```python
from build123d import *

# Parameters (mm, degrees)
BASPROSKE_W        = 9
BASPROSKE_H        = 11
TOOTHCUT_DEPTH     = 18.972200756
TEETHCUTS_COUNT    = 20
TEETHCUTS_ANGLE    = 342
BORSKE_R           = 3.5
BORE_DEPTH         = 50.0000508
SKETCH1_R          = 1.1
CUT_EXTRUDE1_DEPTH = 18.852389344


with BuildPart() as part:
    # BasProSke → Base-Revolve (revolve)
    with BuildSketch(Plane(origin=(0, 0, 0), x_dir=(1, 0, 0), z_dir=(0, 1, 0)), mode=Mode.PRIVATE) as base_revolve_sk:
        with Locations((4.5, 5.5)):
            Rectangle(BASPROSKE_W, BASPROSKE_H)
    revolve(base_revolve_sk.sketch.rotate(Axis((-10, 0, 0), (1, 0, 0)), 180), axis=Axis((-10, 0, 0), (1, 0, 0)))

    # TooCutSke → ToothCut (cut, through all)
    with BuildSketch(Plane(origin=(0, 0, 0), x_dir=(0, 0, -1), z_dir=(1, 0, 0))):
        with BuildLine():
            ThreePointArc((0.499924007, 8.734705318), (0, 8.749), (-0.499924007, 8.734705318))
            ThreePointArc((-0.499924007, 8.734705318), (-0.824302243, 9.905497836), (-1.485192705, 10.924909509))
            ThreePointArc((-1.485192705, 10.924909509), (0, 11.0254), (1.485192705, 10.924909509))
            ThreePointArc((1.485192705, 10.924909509), (0.824302243, 9.905497836), (0.499924007, 8.734705318))
        make_face()
    toothcut = extrude(amount=TOOTHCUT_DEPTH, mode=Mode.SUBTRACT)

    # TeethCuts: ToothCut ×20 about axis
    teethcuts_axis = Axis((-10, 0, 0), (1, 0, 0))
    for i in range(1, TEETHCUTS_COUNT):
        add(toothcut.rotate(teethcuts_axis, i * TEETHCUTS_ANGLE / (TEETHCUTS_COUNT - 1)), mode=Mode.SUBTRACT)

    # BorSke → Bore (cut, symmetric)
    with BuildSketch(Plane(origin=(0, 0, 0), x_dir=(0, 0, -1), z_dir=(1, 0, 0))):
        with Locations(Location((0, 0, 0), (0, 0, 180))):
            Circle(BORSKE_R)
    extrude(amount=BORE_DEPTH, both=True, mode=Mode.SUBTRACT)

    # Sketch1 → Cut-Extrude1 (cut, through all)
    with BuildSketch(Plane(origin=(9, 0, 0), x_dir=(0, 0, -1), z_dir=(1, 0, 0))):
        with Locations((0, -7)):
            Circle(SKETCH1_R)
        with Locations((0, 7)):
            Circle(SKETCH1_R)
        with Locations((7, 0)):
            Circle(SKETCH1_R)
        with Locations((-7, 0)):
            Circle(SKETCH1_R)
    extrude(amount=-CUT_EXTRUDE1_DEPTH, mode=Mode.SUBTRACT)


solid = part.part
```
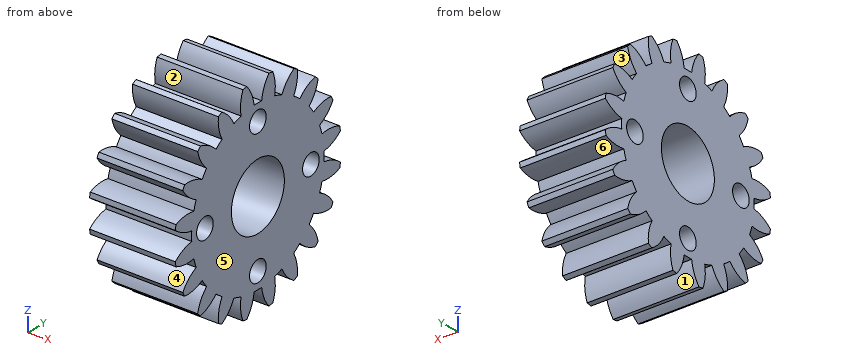
Could you check a few things on this model? Use its own coordinates, in mm. Face numbers are marked on the shaded views. A direction names the side the tool comes from. Round coordinates to 2 decimals unless told otherwise and drop trailing zeros. Write each loop counter-clockwise with the first axis right and the second up, starting at its lowest first coordinate (ties: lowest second). Pieces come first, ordered by that corner, then holes. Notation, with made-up numbers: M 44,9 L 65,9 A12 cw 65,14 Z; hole C 0.25,60 d5. An arc over 180 degrees is marked long. Write each question's results on one line, items separated by ' | '. Start each with the question number.
1. On a 3-axis mill with a long thin cutter (end or side, diameter ignored), from which of +Z, -Z, +X, -X, +Y, -Y can I reach the whole of each face in a straight line? I mean the marked faces 1, 2 and 3. Say none if no direction works.
2. Thinking about a two-plate mould opening in Y: for the marked faces 4, 5 and 6, which applies, +Y half, -Y half, draft (parallel to the pull), parting line (faces both ways), or undercut?
3. I'm going to push flat-ended pins straight in: pin 1 Ø3 at (y, z) = (7, 0) entering from -X; pin 2 Ø2 at (x, z) = (7, 0) entering from +Y; pin 3 Ø2 at (x, z) = (6.5, -8) entering from -Y; pin 4 Ø3 at (x, z) = (6.5, 6.5) entering from -Y. Where does each tip first touch, or does it pass through?
4. Imagine slicing it at A-A on y = 0. List the corners of the cut face in (x, z) for me.
5. I need wall thicknesses on L1, parallel to Y at x = 5, z = 9; L2, parallel to Y at x = 2, z = 0. Which ranges of each line are inside material? Lowest first, please. Write a range as from..to.
6. Imagine slicing it at C-C on x = 2.5. Count the separate pieces of the cut face and the enclosed holes in it, and give its area (3 significant figures).
7. Imagine slicing it at D-D on y = 4. List the corners of the cut face in (x, z) for me, and give its area (3 significant figures).
Result sheet:
1) face 1: -Z, +X, -X | face 2: +X, -X | face 3: +X, -X, +Y
2) face 4: -Y half | face 5: draft | face 6: undercut
3) pin 1: stops at x = 0 | pin 2: stops at y = 10.25 | pin 3: stops at y = -7.96 | pin 4: stops at y = -9.8
4) outline: M 0,-8.75 L 9,-8.75 L 9,-8.1 L 0,-8.1 Z; M 0,-5.9 L 9,-5.9 L 9,-3.5 L 0,-3.5 Z; M 0,3.5 L 9,3.5 L 9,5.9 L 0,5.9 Z; M 0,8.1 L 9,8.1 L 9,8.75 L 0,8.75 Z
5) L1: y = -5.23..-3.7, -2.29..-0.54, 0.54..2.29, 3.7..5.23 | L2: y = -8.75..-8.1, -5.9..-3.5, 3.5..5.9, 8.1..8.75
6) separate pieces: 1 | enclosed holes: 5 | area: 249 mm^2
7) outline: M 0,-9.33 L 9,-9.33 L 9,9.33 L 0,9.33 Z | area: 168 mm^2
